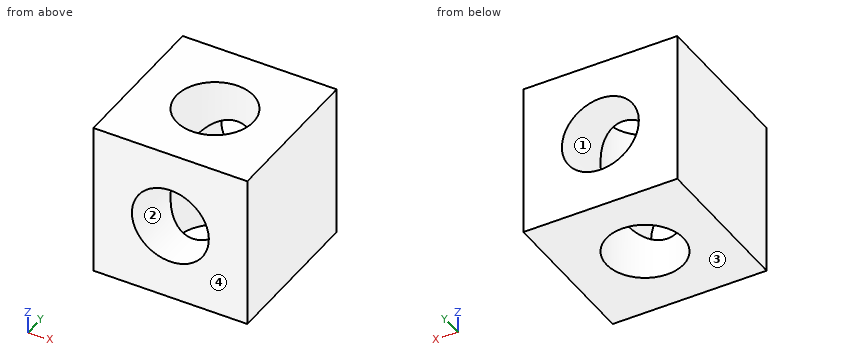
```python
from build123d import *

# Parameters (mm, degrees)
SKETCH_1_W          = 8
SKETCH_1_H          = 8
EXTRUDE_1_DEPTH     = 8
SKETCH_2_R          = 2
CUT_EXTRUDE_1_DEPTH = 22
SKETCH_3_R          = 2
CUT_EXTRUDE_2_DEPTH = 22


with BuildPart() as part:
    # 草图1 → 拉伸1 (new body)
    with BuildSketch(Plane.XY):
        Rectangle(SKETCH_1_W, SKETCH_1_H)
    extrude(amount=EXTRUDE_1_DEPTH)

    # 草图2 → 切除-拉伸1 (cut)
    with BuildSketch(Plane.XY.offset(8)):
        Circle(SKETCH_2_R)
    extrude(amount=-CUT_EXTRUDE_1_DEPTH, mode=Mode.SUBTRACT)

    # 草图3 → 切除-拉伸2 (cut)
    with BuildSketch(Plane(origin=(0, 4, 0), x_dir=(-1, 0, 0), z_dir=(0, 1, 0))):
        with Locations(Location((0, 4, 0), (0, 0, 90))):
            Circle(SKETCH_3_R)
    extrude(amount=-CUT_EXTRUDE_2_DEPTH, mode=Mode.SUBTRACT)


solid = part.part
```
Source: CAD feature listing. Evaluate the final solid. Frame: model axes, mm. Face numbers are marked on the shaded views. Round coordinates to 2 decimals unless told otherwise and drop trailing zeros. Loops run counter-clockwise (first coordinate to the right, second up) from the corner with the lowest first, then second, coordinate; pieces in that order, holes last. Notation, with made-up numbers: M 71,-27.75 L 126,-27.75 A24 ccw 126,-13.75 Z; hole C 10,72.5 d1. An arc over 180 degrees is marked long. Use a Markdown table: item, result. Add a question column.
1. Cut plane A-A, the plane x = 0. Output: boundary loops of the cut face in (y, z).
2. Cut plane B-B, the plane z = 1.5. Output: boundary loops of the cut face in (x, y), and give its area (3 significant figures).
3. Pull-direction query (Z, two-part tool) for the marked faces 1, 2, 3 and 4; classes: +Z half, -Z half, draft (parallel to the pull), parting line (faces both ways), or undercut.
4. Cut plane C-C, the plane y = -1.5. Output: boundary loops of the cut face in (x, z), and give its area (3 significant figures).
5. Cut plane D-D, the plane y = -2.75. Output: boundary loops of the cut face in (x, z).
6. Contact query for a flat-ended pin moving along its axis: pin 1 (3.5 mm diameter, centred on x = 0, z = 4, fed in from -Y). Output: stop coordinate, or through.
7. Ray query, line 1 along X through (y, z) = (-1.45, 4); line 2 along Z through (x, y) = (-0.75, 3.5). Return the intervals inside material, ascending. Write a range as [from, to].
Solution:
| question | item | result |
|---|---|---|
| 1 | outline | M -4,0 L -2,0 L -2,2 L -4,2 Z; M -4,6 L -2,6 L -2,8 L -4,8 Z; M 2,0 L 4,0 L 4,2 L 2,2 Z; M 2,6 L 4,6 L 4,8 L 2,8 Z |
| 2 | outline | M -4,-4 L 4,-4 L 4,4 L -4,4 Z; hole C 0,0 d4 |
| 2 | area | 51.4 mm2 |
| 3 | face 1 | undercut |
| 3 | face 2 | undercut |
| 3 | face 3 | -Z half |
| 3 | face 4 | draft |
| 4 | outline | M -4,0 L -1.32,0 L -1.32,2.5 A2 cw -1.32,5.5 L -1.32,8 L -4,8 Z; M 1.32,0 L 4,0 L 4,8 L 1.32,8 L 1.32,5.5 A2 cw 1.32,2.5 Z |
| 4 | area | 40.0 mm2 |
| 5 | outline | M -4,0 L 4,0 L 4,8 L -4,8 Z; hole C 0,4 d4 |
| 6 | pin 1 | passes through |
| 7 | line 1 | x = [-4, -2], [2, 4] |
| 7 | line 2 | z = [0, 2.15], [5.85, 8] |
